Read the model definition and answer for the solid it produces. Units are mm, in the model's axes. Coordinates: 2 decimals unless noted, no trailing zeros. Answer as a JSON object with one key per item and string values. Group by question number.
from build123d import *

# Parameters (mm, degrees)
F0_R     = 3.175
F1_DEPTH = 76.2
F3_DEPTH = 152.4
F4_W     = 0.508
F4_H     = 149.86
F5_DEPTH = 25.4


with BuildPart() as f1:
    # F0 (on Top) → F1 (new body, symmetric)
    with BuildSketch(Plane.XY):
        Circle(F0_R)
    extrude(amount=F1_DEPTH, both=True)

    # F2 (on face) → F3 (cut)
    with BuildSketch(Plane.XY.offset(76.2)):
        with BuildLine():
            Line((2.3540518227, -2.1305081591), (-2.7044223431, -1.6633474653))
            ThreePointArc((-2.7044223431, -1.6633474653), (-0.2919754336, -3.1615463536), (2.3540518227, -2.1305081591))
        make_face()
    extrude(amount=-F3_DEPTH, mode=Mode.SUBTRACT)

    # F4 (on face) → F5 (cut)
    with BuildSketch(Plane(origin=(-0.1751852602, -1.8969278122, 0), x_dir=(0.9957626311, -0.0919607665, 0), z_dir=(-0.0919607665, -0.9957626311, 0))):
        Rectangle(F4_W, F4_H)
        with BuildLine():
            Line((0.254, -74.93), (-0.254, -74.93))
            ThreePointArc((-0.254, -74.93), (0, -75.184), (0.254, -74.93))
        make_face()
        with BuildLine():
            ThreePointArc((0.254, 74.93), (0, 75.184), (-0.254, 74.93))
            Line((-0.254, 74.93), (0.254, 74.93))
        make_face()
    extrude(amount=-F5_DEPTH, mode=Mode.SUBTRACT)


solid = f1.part
1. For a pull along X with two mould halves and no side action, classify faces 1 (the flat face through (0, 1, -76.2)), 2 (the cylindrical face through (-1.15, 2.96, 1.07)), 3 (the flat face through (0.308, 0.569, -1.049)) as pulls with the +X half, pulls with the -X half, needs draft (parallel to the pull), parting line crosses it, or undercut.
2. Straight lines are drawn through the part: L1, parallel to Z at x = 0.25, y = 1.9; L2, parallel to X at y = 2.65, z = 31; L3, parallel to Z at x = 0, y = 2.35. For each, find the intervals that lie inside material, in ascending order.
3. Given pin 1 (2 mm diameter, centred on x = -1.5, z = -42, fed in from -Y), flat-ended and moving along its own axis, determine where the tip first touches the part or whether it passes through.
Derived:
{
 "1": {"face 1": "needs draft", "face 2": "parting line crosses it", "face 3": "undercut"},
 "2": {"L1": "z = -76.2 to -75.17, 75.17 to 76.2", "L2": "x = -1.75 to -0.01, 0.5 to 1.75", "L3": "z = -76.2 to -75.06, 75.06 to 76.2"},
 "3": {"pin 1": "stops at y = -1.87"}
}
